```python
from build123d import *
from build123d.topology import SkipClean

# Parameters (mm, degrees)
SKETCH2_R                = 60
BOSS_EXTRUDE1_DEPTH      = 60
SKETCH3_W                = 10
SKETCH3_H                = 10.47851478
BOSS_EXTRUDE2_DEPTH      = 60
FILLET2_R                = 3
CIRPATTERN1_COUNT        = 18
FILLET2_OF_CIRPATTERN1_R = 3
SKETCH4_R                = 10
CUT_EXTRUDE1_DEPTH       = 60
SKETCH5_R                = 22.481820488
BOSS_EXTRUDE3_DEPTH      = 60
SKETCH6_R                = 12.5
CUT_EXTRUDE2_DEPTH       = 12
CUT_EXTRUDE3_DEPTH       = 30.5
SCALE1_SCALE             = 0.2


with BuildPart() as part:
    # Sketch2 → Boss-Extrude1 (new body)
    with BuildSketch(Plane.XY):
        Circle(SKETCH2_R)
    extrude(amount=BOSS_EXTRUDE1_DEPTH)

    # Sketch3 → Boss-Extrude2 (add)
    with BuildSketch(Plane.XY.offset(60)):
        with Locations((0, 64.76074261)):
            Rectangle(SKETCH3_W, SKETCH3_H)
    boss_extrude2 = extrude(amount=-BOSS_EXTRUDE2_DEPTH)

    # Fillet2
    fillet2_edges = [part.edges().sort_by_distance(p)[0] for p in [
        (5, 70, 30),
        (0, 70, 0),
        (-5, 70, 30),
        (0, 70, 60),
    ]]
    fillet(fillet2_edges, radius=FILLET2_R)

    # CirPattern1: Boss-Extrude2 ×18 about axis
    cirpattern1_axis = Axis((0, 0, 0), (0, 0, 1))
    for i in range(1, CIRPATTERN1_COUNT):
        add(boss_extrude2.rotate(cirpattern1_axis, i * 360 / CIRPATTERN1_COUNT))

    # Fillet2 of CirPattern1
    fillet2_of_cirpattern1_edges = [part.edges().sort_by_distance(p)[0] for p in [
        (-19.242946929, 67.488584172, 30),
        (-23.941410033, 65.778483455, 0),
        (-28.639873137, 64.068382738, 30),
        (-23.941410033, 65.778483455, 60),
        (-41.164910462, 56.837049067, 30),
        (-44.995132678, 53.623111018, 0),
        (-48.825354894, 50.40917297, 30),
        (-44.995132678, 53.623111018, 60),
        (-58.121778265, 39.330127019, 30),
        (-60.621778265, 35, 0),
        (-63.121778265, 30.669872981, 30),
        (-60.621778265, 35, 60),
        (-68.068301823, 17.079411202, 30),
        (-68.936542711, 12.155372437, 0),
        (-69.804783599, 7.231333672, 30),
        (-68.936542711, 12.155372437, 60),
        (-69.804783599, -7.231333672, 30),
        (-68.936542711, -12.155372437, 0),
        (-68.068301823, -17.079411202, 30),
        (-68.936542711, -12.155372437, 60),
        (-63.121778265, -30.669872981, 30),
        (-60.621778265, -35, 0),
        (-58.121778265, -39.330127019, 30),
        (-60.621778265, -35, 60),
        (-48.825354894, -50.40917297, 30),
        (-44.995132678, -53.623111018, 0),
        (-41.164910462, -56.837049067, 30),
        (-44.995132678, -53.623111018, 60),
        (-28.639873137, -64.068382738, 30),
        (-23.941410033, -65.778483455, 0),
        (-19.242946929, -67.488584172, 30),
        (-23.941410033, -65.778483455, 60),
        (-5, -70, 30),
        (0, -70, 0),
        (5, -70, 30),
        (0, -70, 60),
        (19.242946929, -67.488584172, 30),
        (23.941410033, -65.778483455, 0),
        (28.639873137, -64.068382738, 30),
        (23.941410033, -65.778483455, 60),
        (41.164910462, -56.837049067, 30),
        (44.995132678, -53.623111018, 0),
        (48.825354894, -50.40917297, 30),
        (44.995132678, -53.623111018, 60),
        (58.121778265, -39.330127019, 30),
        (60.621778265, -35, 0),
        (63.121778265, -30.669872981, 30),
        (60.621778265, -35, 60),
        (68.068301823, -17.079411202, 30),
        (68.936542711, -12.155372437, 0),
        (69.804783599, -7.231333672, 30),
        (68.936542711, -12.155372437, 60),
        (69.804783599, 7.231333672, 30),
        (68.936542711, 12.155372437, 0),
        (68.068301823, 17.079411202, 30),
        (68.936542711, 12.155372437, 60),
        (63.121778265, 30.669872981, 30),
        (60.621778265, 35, 0),
        (58.121778265, 39.330127019, 30),
        (60.621778265, 35, 60),
        (48.825354894, 50.40917297, 30),
        (44.995132678, 53.623111018, 0),
        (41.164910462, 56.837049067, 30),
        (44.995132678, 53.623111018, 60),
        (28.639873137, 64.068382738, 30),
        (23.941410033, 65.778483455, 0),
        (19.242946929, 67.488584172, 30),
        (23.941410033, 65.778483455, 60),
    ]]
    fillet(fillet2_of_cirpattern1_edges, radius=FILLET2_OF_CIRPATTERN1_R)

    # Sketch4 → Cut-Extrude1 (cut)
    with BuildSketch(Plane.XY.offset(60)):
        Circle(SKETCH4_R)
    extrude(amount=-CUT_EXTRUDE1_DEPTH, mode=Mode.SUBTRACT)

    # Sketch5 → Boss-Extrude3 (add)
    with BuildSketch(Plane.XY.offset(60)):
        Circle(SKETCH5_R)
    extrude(amount=-BOSS_EXTRUDE3_DEPTH)

    # Sketch6 → Cut-Extrude2 (cut)
    with BuildSketch(Plane.XY.offset(60)):
        Circle(SKETCH6_R)
    extrude(amount=-CUT_EXTRUDE2_DEPTH, mode=Mode.SUBTRACT)

    # Sketch7 → Cut-Extrude3 (cut)
    with SkipClean():  # the faces are left unmerged after this step: merging them gives an invalid solid
        with BuildSketch(Plane.XY.offset(48)):
            with BuildLine():
                Line((10.037305415, -7.45), (-10.037305415, -7.45))
                ThreePointArc((-10.037305415, -7.45), (-12.5, 0), (-10.037305415, 7.45))
                Line((-10.037305415, 7.45), (10.037305415, 7.45))
                ThreePointArc((10.037305415, 7.45), (12.5, 0), (10.037305415, -7.45))
            make_face()
        extrude(amount=-CUT_EXTRUDE3_DEPTH, mode=Mode.SUBTRACT)


with BuildPart() as part_1:
    # Scale1: scaled about (3e-09, 1e-09, 29.777250978)
    add(part.part.scale(SCALE1_SCALE).moved(Location((2e-09, 1e-09, 23.821800782))))


solid = part_1.part
```
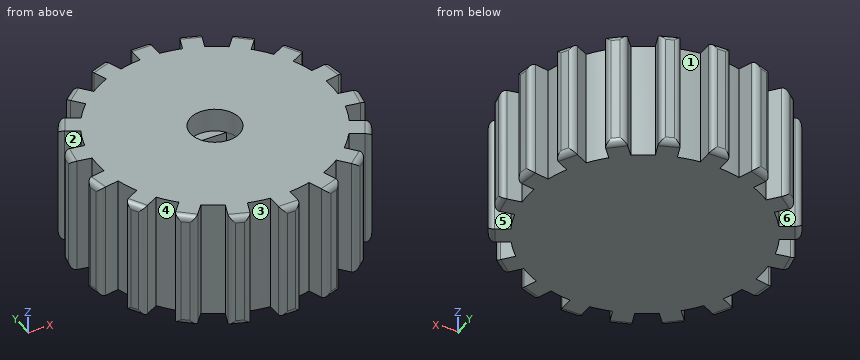
Read the model definition and answer for the solid it produces. Units are mm, in the model's axes. Face numbers are marked on the shaded views. A direction names the side the tool comes from. Give positions to 0.01 mm unless a question says otherwise; leave off trailing zeros. Order: outer loops, then holes, each group sorted by start corner. A loop starts at its lowest first (then second) coordinate and runs counter-clockwise, first axis right, second up. Notation, with made-up numbers: (39, 36) -> (86, 36) arc R26 ccw to (86, 59) -> close; hole circle Ø1 at (8, -40). An arc over 180 degrees is marked (long way). Write item = value, one per line.
1. A cutting plane is placed at B-B, the plane y = 0. Write down the section's boundary in (x, z).
Numbers:
outline = (-12, 23.82) -> (12, 23.82) -> (12, 35.82) -> (2.5, 35.82) -> (2.5, 27.32) -> (-2.5, 27.32) -> (-2.5, 35.82) -> (-12, 35.82) -> close
2. The mould has two halves that part along Y. Classify the marked faces 1, 2 and 3: +Y half, -Y half, draft (parallel to the pull), parting line (faces both ways), or undercut.
Numbers:
face_1 = +Y half
face_2 = undercut
face_3 = -Y half
3. A cutting plane is placed at C-C, the plane y = -3.75. Write down the section's boundary in (x, z).
Numbers:
outline = (-11.4, 23.82) -> (11.4, 23.82) -> (11.4, 35.82) -> (-11.4, 35.82) -> close
4. Straight lines are drawn through the part: line 1 along Y through (x, z) = (0, 34.3); line 2 along X through (y, z) = (10.5, 26.5); line 3 along X through (y, z) = (-10.75, 25.25). For each, find the intervals that lie inside material, in ascending order.
Numbers:
line_1 = -14 to -2.5, 2.5 to 14
line_2 = -9.27 to -7.51, -5.81 to 5.81, 7.51 to 9.27
line_3 = -8.97 to -7.71, -5.33 to 5.33, 7.71 to 8.97
5. A cutting plane is placed at A-A, the plane x = 0. Write down the section's boundary in (y, z).
Numbers:
outline = (-14, 24.42) arc R0.6 ccw to (-13.4, 23.82) -> (13.4, 23.82) arc R0.6 ccw to (14, 24.42) -> (14, 35.22) arc R0.6 ccw to (13.4, 35.82) -> (2.5, 35.82) -> (2.5, 33.42) -> (1.49, 33.42) -> (1.49, 27.32) -> (-1.49, 27.32) -> (-1.49, 33.42) -> (-2.5, 33.42) -> (-2.5, 35.82) -> (-13.4, 35.82) arc R0.6 ccw to (-14, 35.22) -> close
6. Given pin 1 (1.2 mm diameter, centred on y = 12.5, z = 30, fed in from -X); pin 2 (1.6 mm diameter, centred on y = -12.5, z = 29.5, fed in from +X); pin 3 (4 mm diameter, centred on x = 0, y = 0, fed in from +Z), each flat-ended and moving along its own axis, determine where each tip first touches the part or whether it passes through.
Numbers:
pin_1 = -5.56
pin_2 = 5.56
pin_3 = 33.42
7. For the marked faces 4, 5 and 6, determine the directions among +Z, -Z, +X, -X, +Y, -Y from which every point of the face is accessible in a straight line to the end or side of a thin tool.
Numbers:
face_4 = +Z, -Z
face_5 = +Z, -Z, +X
face_6 = +Z, -Z, +Y
